from build123d import *

# Parameters (mm, degrees)
F0_W     = 273.05
F0_H     = 114.3
F1_DEPTH = 19.05
F2_R     = 25.4
F3_DEPTH = 25.4
F5_DEPTH = 25.4
F7_DEPTH = 25.4


with BuildPart() as f1:
    # F0 (on Front) → F1 (new body)
    with BuildSketch(Plane.XZ):
        with Locations((136.525, 57.15)):
            Rectangle(F0_W, F0_H)
    extrude(amount=F1_DEPTH)

    # F2 (on face) → F3 (cut)
    with BuildSketch(Plane.XZ.offset(19.05)):
        with Locations((50.8, 50.8)):
            Circle(F2_R)
        with Locations((222.25, 50.8)):
            Circle(F2_R)
    extrude(amount=-F3_DEPTH, mode=Mode.SUBTRACT)

    # F4 (on face) → F5 (cut)
    with BuildSketch(Plane.XZ.offset(19.05)):
        with BuildLine():
            Line((177.8, 114.3), (95.25, 114.3))
            Line((95.25, 114.3), (95.25, 53.975))
            ThreePointArc((95.25, 53.975), (98.039808, 47.239808), (104.775, 44.45))
            Line((104.775, 44.45), (168.275, 44.45))
            ThreePointArc((168.275, 44.45), (175.010192, 47.239808), (177.8, 53.975))
            Line((177.8, 53.975), (177.8, 114.3))
        make_face()
    extrude(amount=-F5_DEPTH, mode=Mode.SUBTRACT)

    # F6 (on face) → F7 (cut)
    with BuildSketch(Plane.XZ.offset(19.05)):
        Polygon((71.372664, 35.902836), (49.335122, 25.442277), (223.714878, 25.442277), (201.677336, 35.902836), (161.071733, 35.902836), (161.071733, 44.45), (141.377911, 44.45), (141.377911, 35.902836), align=None)
    extrude(amount=-F7_DEPTH, mode=Mode.SUBTRACT)


solid = f1.part
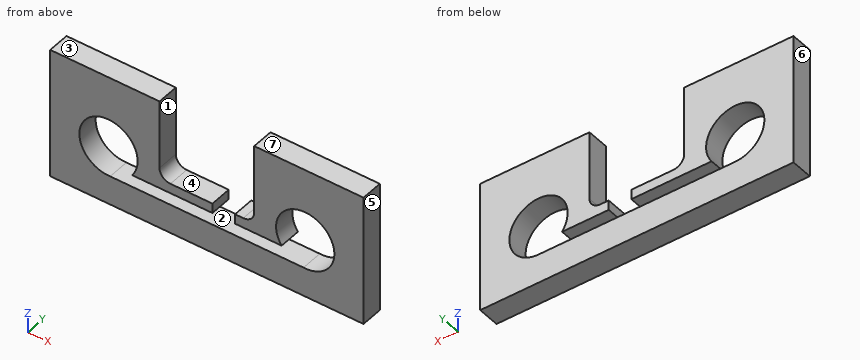
Input: part model. Units: mm. Frame: model coordinates. Face numbers are marked on the shaded views. A direction names the side the tool comes from. Coordinates: 2 decimals unless noted, no trailing zeros. Loops run counter-clockwise (first coordinate to the right, second up) from the corner with the lowest first, then second, coordinate; pieces in that order, holes last. Notation, with made-up numbers: (-25.5, 21) - (13.5, 21) arc R22 ccw to (13.5, 40) - close; hole circle Ø2 at (69, -8). An arc over 180 degrees is marked (long way). Answer in a Markdown table with one row per item. Add a question column.
Item 1: Section query B-B on y = -10.25. Return the cut outline in (x, z) (3 decimals).
Item 2: Line query: line 1 along X through (y, z) = (-10, 91.5); line 2 along X through (y, z) = (-4.25, 50.8); line 3 along X through (y, z) = (-13.75, 66). Output: solid intervals per line, ascending. Write a range as [from, to].
Item 3: Section query A-A on x = 122.5. Return the cut outline in (y, z), then the cut area to 4 significant figures.
Item 4: Access query for the marked faces 1, 2 and 3. Directions: +Z, -Z, +X, -X, +Y, -Y. A direction counts if a zero-diameter tool reaches every point of the face in a straight line with its end or side. Return the directions, or none.
Item 5: Mould query, pull axis X, two halves, no side actions, for the marked faces 4, 5, 6 and 7. Classes: released by +X, released by -X, zero draft, split by the parting line, or undercut.
Item 6: Section query D-D on x = 89.5. Return the cut outline in (y, z).
Item 7: Section query C-C on z = 47.5. Return the cut outline in (x, y), then the cut area to 3 significant figures.
Item 8: Contact query for flat-ended pins moving along their axis: P1, Ø5.5, axis at x = 186, y = -6.5, coming from the -Z side; P2, Ø8, axis at x = 164, y = -14, coming from the +Z side. Output: stop coordinate, or through.
Recorded:
| question | item | result |
|---|---|---|
| 1 | outline | (0, 0) - (273.05, 0) - (273.05, 114.3) - (177.8, 114.3) - (177.8, 53.975) arc R9.525 cw to (168.275, 44.45) - (161.072, 44.45) - (161.072, 35.903) - (201.677, 35.903) arc R25.4 cw (long way) to (220.785, 25.442) - (52.265, 25.442) arc R25.4 cw (long way) to (71.373, 35.903) - (141.378, 35.903) - (141.378, 44.45) - (104.775, 44.45) arc R9.525 cw to (95.25, 53.975) - (95.25, 114.3) - (0, 114.3) - close |
| 2 | line 1 | [0, 95.25], [177.8, 273.05] |
| 2 | line 2 | [0, 25.4], [76.2, 95.79], [177.26, 196.85], [247.65, 273.05] |
| 2 | line 3 | [0, 30.45], [71.15, 95.25], [177.8, 201.9], [242.6, 273.05] |
| 3 | outline | (-19.05, 0) - (0, 0) - (0, 25.44) - (-19.05, 25.44) - close; (-19.05, 35.9) - (0, 35.9) - (0, 44.45) - (-19.05, 44.45) - close |
| 3 | area | 647.5 mm^2 |
| 4 | face 1 | +Z, +Y, -Y |
| 4 | face 2 | +Y, -Y |
| 4 | face 3 | +Z, +X, -X, +Y, -Y |
| 5 | face 4 | undercut |
| 5 | face 5 | released by +X |
| 5 | face 6 | released by -X |
| 5 | face 7 | zero draft |
| 6 | outline | (-19.05, 0) - (0, 0) - (0, 25.44) - (-19.05, 25.44) - close; (-19.05, 35.9) - (0, 35.9) - (0, 114.3) - (-19.05, 114.3) - close |
| 7 | outline | (0, -19.05) - (25.62, -19.05) - (25.62, 0) - (0, 0) - close; (75.98, -19.05) - (97.79, -19.05) - (97.79, 0) - (75.98, 0) - close; (175.26, -19.05) - (197.07, -19.05) - (197.07, 0) - (175.26, 0) - close; (247.43, -19.05) - (273.05, -19.05) - (273.05, 0) - (247.43, 0) - close |
| 7 | area | 1,810 mm^2 |
| 8 | P1 | z = 0 |
| 8 | P2 | z = 44.45 |
